Model file for the job. Use its own axes, mm. A direction names the side the tool comes from. Give positions to 0.01 mm unless a question says otherwise; leave off trailing zeros. Order: outer loops, then holes, each group sorted by start corner. A loop starts at its lowest first (then second) coordinate and runs counter-clockwise, first axis right, second up. Notation, with made-up numbers: (-16, 6) - (6, 6) arc R32 cw to (6, 42) - close; hole circle Ø11 at (38.25, 63). An arc over 180 degrees is marked (long way). Use CSV: the item, a comma, the result in double quotes. Start each with the question number.
(1) Tool access for faces 4 (the flat face through (5, 1.15, 17)), 5 (the flat face through (5, -6, 13.57)), 6 (the flat face through (9.03, 2.12, 16.61)), 7 (the flat face through (5, 5.1, 17)): list every direction of +Z, -Z, +X, -X, +Y, -Y with a clear straight run to the whole face (end or side of a thin tool).
(2) Band-saw the part on C-C, the plane y = -6. Give the cut face in (x, z), then the cut area to 3 significant figures.
(3) Drop flat-ended pins along their axis: pin 1 Ø2 at (x, z) = (6, 17) entering from +Y; pin 2 Ø2 at (x, y) = (3.5, 3.5) entering from +Z; pin 3 Ø1.5 at (x, y) = (8, 2) entering from -Z. Give the stop position or say it passes through.
(4) Pull direction Z, two halves, no side cores. Call faces 1 (the flat face through (4.93, 4.095, 5.422)), 2 (the flat face through (5, -1, 13.57)), 3 (the cylindrical face through (4.93, -1.514, 6.123)): +Z half, -Z half, draft (parallel to the pull), parting line (faces both ways), or undercut.
(5) Band-saw the part on B-B, the plane y = -1. Give the cut face in (x, z) (3 decimals).
(6) Band-saw the part on D-D, the plane x = 1.75. Give the cut face in (y, z).
(7) Band-saw the part on A-A, the plane z = 18.5. Give the cut face in (x, y) (3 decimals), then the cut area to 3 significant figures.
(8) Probe L1, parallel to Y at x = 4.75, z = 20.5; L2, parallel to Z at x = 8, y = -6; L3, parallel to Z at x = 4, y = -6.25. List the from-to ranges inside material, lowest first.
from build123d import *

# Parameters (mm, degrees)
BOSS_EXTRUDE1_DEPTH = 10
BOSS_EXTRUDE4_DEPTH = 9
BOSS_EXTRUDE5_DEPTH = 9


with BuildPart() as part:
    # Sketch1 → Boss-Extrude1 (new body)
    with BuildSketch(Plane(origin=(0, 0, 0), x_dir=(0, 0, -1), z_dir=(1, 0, 0))):
        with BuildLine():
            Line((-8.569568251, -0.25), (-13.569568251, -0.25))
            Line((-13.569568251, -0.25), (-13.569568251, -6.5))
            Line((-13.569568251, -6.5), (-9.398337093, -3.25))
            ThreePointArc((-9.398337093, -3.25), (-8.248911648, -3.193857851), (-7.80775466, -4.256736633))
            ThreePointArc((-7.80775466, -4.256736633), (4.148003929, -12.840618642), (2.063858472, 1.729197126))
            ThreePointArc((2.063858472, 1.729197126), (1.600092206, 1.859034064), (1.13958663, 2))
            Line((1.13958663, 2), (-12.169568251, 6.25))
            Line((-12.169568251, 6.25), (-12.169568251, 0))
            Line((-12.169568251, 0), (0, 0))
            ThreePointArc((0, 0), (3.535533906, -10.847679857), (-5.7130455, -4.166666667))
            ThreePointArc((-5.7130455, -4.166666667), (-6.145728322, -1.482233047), (-8.569568251, -0.25))
        make_face()
    extrude(amount=BOSS_EXTRUDE1_DEPTH)

    # Sketch2 → Boss-Extrude4 (add)
    with BuildSketch(Plane.XY.offset(12.169568251)):
        Polygon((0, 1.15), (10, 1.15), (8.025, 3.125), (10, 5.1), (0, 5.1), align=None)
    extrude(amount=BOSS_EXTRUDE4_DEPTH)

    # Sketch3 → Boss-Extrude5 (add)
    with BuildSketch(Plane.XY.offset(13.569568251)):
        Polygon((0, -5.35), (10, -5.35), (8.025, -3.375), (10, -1.4), (0, -1.4), align=None)
    extrude(amount=BOSS_EXTRUDE5_DEPTH)


solid = part.part
Answer block:
1,face 4,"+Z, +X, -X"
1,face 5,"+Z, +X, -X, -Y"
1,face 6,"+Z, +X"
1,face 7,"+Z, +X, -X, +Y"
2,outline,"(0, -8) - (10, -8) - (10, -6) - (0, -6) - close; (0, 6) - (10, 6) - (10, 8) - (0, 8) - close; (0, 12.93) - (10, 12.93) - (10, 13.57) - (0, 13.57) - close"
2,area,"46.4 mm2"
3,pin 1,"stops at y = 5.1"
3,pin 2,"stops at z = 21.17"
3,pin 3,"stops at z = -3.38"
4,face 1,"-Z half"
4,face 2,"+Z half"
4,face 3,"undercut"
5,outline,"(0, -6.245) - (10, -6.245) - (10, -3.317) - (0, -3.317) - close; (0, 6.585) - (10, 6.585) - (10, 13.57) - (0, 13.57) - close"
6,outline,"(-6.5, 13.57) - (-3.25, 9.4) arc R1 cw to (-4.26, 7.81) arc R8 ccw (long way) to (1.73, -2.06) arc R20 cw to (2, -1.14) - (6.25, 12.17) - (5.1, 12.17) - (5.1, 21.17) - (1.15, 21.17) - (1.15, 12.17) - (0, 12.17) - (0, 0) arc R6 cw (long way) to (-4.17, 5.71) arc R3 ccw to (-0.25, 8.57) - (-0.25, 13.57) - (-1.4, 13.57) - (-1.4, 22.57) - (-5.35, 22.57) - (-5.35, 13.57) - close"
7,outline,"(0, -5.35) - (10, -5.35) - (8.025, -3.375) - (10, -1.4) - (0, -1.4) - close; (0, 1.15) - (10, 1.15) - (8.025, 3.125) - (10, 5.1) - (0, 5.1) - close"
7,area,"71.2 mm2"
8,L1,"y = -5.35 to -1.4, 1.15 to 5.1"
8,L2,"z = -8 to -6, 6 to 8, 12.93 to 13.57"
8,L3,"z = -8 to -5.99, 5.99 to 8, 13.25 to 13.57"
